from build123d import *

# Parameters (mm, degrees)
SKETCH1_R           = 10.75
SKETCH1_R_2         = 8
BOSS_EXTRUDE1_DEPTH = 2.7
CHAMFER1_SIZE       = 0.5
CHAMFER1_SIZE2      = 1.866025404
CHAMFER2_SIZE       = 2
CHAMFER2_SIZE2      = 0.535898385
SKETCH3_OUTSIDE_W   = 29.606
SKETCH3_OUTSIDE_H   = 29.606
CUT_EXTRUDE1_DEPTH  = 2.7


with BuildPart() as part:
    # Sketch1 → Boss-Extrude1 (new body)
    with BuildSketch(Plane(origin=(0, 0, 0), x_dir=(1, 0, 0), z_dir=(0, 1, 0))):
        with Locations(Location((0, 0, 0), (0, 0, 90))):
            Circle(SKETCH1_R)
        with Locations(Location((0, 0, 0), (0, 0, 90))):
            Circle(SKETCH1_R_2, mode=Mode.SUBTRACT)
    extrude(amount=BOSS_EXTRUDE1_DEPTH)

    # Chamfer1
    chamfer1_edges = [part.edges().sort_by_distance(p)[0] for p in [
        (0, 2.7, 10.75),
    ]]
    chamfer1_side = [part.faces().sort_by_distance(p)[0] for p in [
        (0, 1.35, 10.75),
    ]]
    chamfer(chamfer1_edges, length=CHAMFER1_SIZE, length2=CHAMFER1_SIZE2, reference=chamfer1_side[0])

    # Chamfer2
    chamfer2_edges = [part.edges().sort_by_distance(p)[0] for p in [
        (0, 0, 10.75),
    ]]
    chamfer2_side = [part.faces().sort_by_distance(p)[0] for p in [
        (0, 0, 10.445944084),
    ]]
    chamfer(chamfer2_edges, length=CHAMFER2_SIZE, length2=CHAMFER2_SIZE2, reference=chamfer2_side[0])

    # Sketch3 outside → Cut-Extrude1 (cut)
    with BuildSketch(Plane(origin=(0, 2.7, 0), x_dir=(1, 0, 0), z_dir=(0, 1, 0))):
        Rectangle(SKETCH3_OUTSIDE_W, SKETCH3_OUTSIDE_H)
        Polygon((0, 10.854185061), (-9.4, 5.42709253), (-9.4, -5.42709253), (0, -10.854185061), (9.4, -5.42709253), (9.4, 5.42709253), align=None, mode=Mode.SUBTRACT)
    extrude(amount=-CUT_EXTRUDE1_DEPTH, mode=Mode.SUBTRACT)


solid = part.part
Geometry check sheet. Reference: the model listing, model coordinates, mm. Coordinates: 2 decimals unless noted, no trailing zeros. Order: outer loops, then holes, each group sorted by start corner. A loop starts at its lowest first (then second) coordinate and runs counter-clockwise, first axis right, second up. Notation, with made-up numbers: (-4.5, -19) - (32.5, -19) arc R26 ccw to (32.5, 10) - close; hole circle Ø5 at (30.25, 47.25). An arc over 180 degrees is marked (long way). Answer in a Markdown table with one row per item. Add a question column.
1) Release check for a two-part mould opening along X. For faces 1 (the flat face through (9.4, 1, 0)), 2 (the cylindrical face through (7.81, 1.33, 1.73)), 3 (the flat face through (-9.4, 1, 0)), 4 (the flat face through (3, 0, -8)) record: +X half, -X half, draft (parallel to the pull), parting line (faces both ways), or undercut.
2) Material ranges on line 1 along Z through (x, y) = (2, 2.4); line 2 along Y through (x, z) = (0.5, 8.75); line 3 along Z through (x, y) = (1.5, 1.05), recorded low to high. Write a range as [from, to].
3) Cross-section at B-B, the plane y = 1.3. Record the cut outline in (x, z), then the cut area to 3 significant figures.
4) Gauge pin test, flat ends, axial feed: P1, Ø5, axis at x = -0.5, z = 5, coming from the -Y side; P2, Ø1, axis at x = -7.5, y = 2, coming from the +Z side; P3, Ø1, axis at x = 5.5, y = 1, coming from the -Z side. Record the tip position at first contact, or that the pin passes through.
5) Cross-section at A-A, the plane z = 0. Record the cut outline in (x, y), then the cut area to 3 significant figures.
Check result:
| question | item | result |
|---|---|---|
| 1 | face 1 | +X half |
| 1 | face 2 | undercut |
| 1 | face 3 | -X half |
| 1 | face 4 | draft |
| 2 | line 1 | z = [-9.7, -7.75], [7.75, 9.7] |
| 2 | line 2 | y = [0, 2.7] |
| 2 | line 3 | z = [-9.99, -7.86], [7.86, 9.99] |
| 3 | outline | (-9.4, -5.22) arc R10.75 ccw to (-9.22, -5.53) - (-0.18, -10.75) arc R10.75 ccw to (0.18, -10.75) - (9.22, -5.53) arc R10.75 ccw to (9.4, -5.22) - (9.4, 5.22) arc R10.75 ccw to (9.22, 5.53) - (0.18, 10.75) arc R10.75 ccw to (-0.18, 10.75) - (-9.22, 5.53) arc R10.75 ccw to (-9.4, 5.22) - close; hole circle Ø16 at (0, 0) |
| 3 | area | 105 mm² |
| 4 | P1 | passes through |
| 4 | P2 | stops at z = 6.81 |
| 4 | P3 | stops at z = -7.97 |
| 5 | outline | (-9.4, 0.17) - (-8.75, 0) - (-8, 0) - (-8, 2.7) - (-8.88, 2.7) - (-9.4, 2.56) - close; (8, 0) - (8.75, 0) - (9.4, 0.17) - (9.4, 2.56) - (8.88, 2.7) - (8, 2.7) - close |
| 5 | area | 7.38 mm² |
